Autodesk Inventor part; units mm, degrees
ref_plane "YZ Plane" through (0, 0, 0) normal (1, 0, 0) x (0, 1, 0)
ref_plane "XZ Plane" through (0, 0, 0) normal (0, 1, 0) x (-1, 0, 0)
ref_plane "XY Plane" through (0, 0, 0) normal (0, 0, 1) x (1, 0, 0)
sketch "Sketch1" plane through (0, 0, 0) normal (0, 0, 1) x (1, 0, 0)
  circle A0 centre (0, 0) radius 4
  line L0 (-10, -10) -> (10, -10)
  line L1 (10, -10) -> (10, 10)
  line L2 (10, 10) -> (-10, 10)
  line L3 (-10, 10) -> (-10, -10)
  line L4 (-10, -10) -> (10, 10) construction
  line L5 (10, -10) -> (-10, 10) construction
  dimension "d0" = 8
  dimension "d3" = 20
  dimension "d4" = 10
  dimension "d5" = 10
extrude "Extrusion1" add sketch "Sketch1" along normal blind 30 and the other way blind 20
extrude "Extrusion2" add sketch "Sketch1" against normal up to surface (20 mm away) contours A0
sketch "Sketch2" plane through (-10, -10, 30) normal (-1, 0, 0) x (0, 0, 1)
  line L0 (-50, 20) -> (-50, 0)
  line L1 (-50, 20) -> (-30, 20)
  line L2 (-30, 20) -> (-30, 0)
  line L3 (-30, 0) -> (-50, 0)
  line L4 (-50, 0) -> (-50, 20)
  point P0 (-30, 10)
extrude "Extrusion3" add sketch "Sketch2" along normal blind 30
sketch "Sketch3" plane through (-10, -10, 30) normal (0, -1, 0) x (1, 0, 0)
  line L0 (0, -30) -> (-30, -30)
  line L1 (0, -30) -> (20, -30)
  line L2 (20, -30) -> (20, -50)
  line L3 (20, -50) -> (0, -50)
  line L4 (0, -50) -> (0, -30)
  point P0 (10, -30)
extrude "Extrusion4" add sketch "Sketch3" along normal blind 30
sketch "Sketch4" plane through (-40, -10, 30) normal (-1, 0, 0) x (0, 0, 1)
  circle A0 centre (-40, 10) radius 4
  point P0 (-30, 10)
  dimension "d16" = 8
extrude "Extrusion5" cut sketch "Sketch4" against normal blind 30
sketch "Sketch5" plane through (-10, -40, 30) normal (0, -1, 0) x (1, 0, 0)
  circle A0 centre (10, -40) radius 4
  point P0 (10, -30)
  dimension "d19" = 8
extrude "Extrusion6" cut sketch "Sketch5" against normal blind 30
sketch "Sketch6" plane through (0, 0, -20) normal (0, 0, -1) x (-1, 0, 0)
  line L0 (10, -10) -> (40, -10)
  line L1 (10, -10) -> (10, -40)
  line L2 (10, -40) -> (-10, -40)
  line L3 (40, -10) -> (10, -40)
  point P0 (0, 0)
extrude "Extrusion7" add sketch "Sketch6" against normal blind 20
sketch "Sketch7" plane through (-10, 10, 30) normal (0, 1, 0) x (1, 0, 0)
  line L0 (-30, 30) -> (-30, 50)
  line L1 (0, 30) -> (-30, 30)
  line L2 (-30, 30) -> (0, 30)
  line L3 (0, 0) -> (20, 0)
  line L4 (0, 30) -> (0, 0)
  line L5 (0, 0) -> (-30, 30)
  point P0 (10, 30)
extrude "Extrusion8" add sketch "Sketch7" against normal blind 20
sketch "Sketch8" plane through (10, -10, 30) normal (1, 0, 0) x (0, 0, -1)
  line L0 (30, 0) -> (0, 0)
  line L1 (30, 0) -> (30, -30)
  line L2 (0, 20) -> (0, 0)
  line L3 (0, 0) -> (30, -30)
  point P0 (30, 10)
extrude "Extrusion9" add sketch "Sketch8" against normal blind 20
sketch "Sketch9" plane through (10, 10, 30) normal (0, 1, 0) x (1, 0, 0)
  line L0 (-50, 36) -> (-20, 36)
  line L1 (-14, 30) -> (-14, 0)
  circle A0 centre (-26.3015, 23.6985) radius 12.3015
  line L2 (-50, 30) -> (-20, 0)
  point P0 (-10, 30)
hole "Hole1" at (-16.3015, 10, 6.3015) direction (0, -1, 0) diameter 3.5 end through all
fillet "Fillet1" radius 4 3 edges at (-10, -25, 0) (-10, -10, 15) (-25, -10, 0)
fillet "Fillet2" radius 4 1 edges at (10, -15, -20)
fillet "Fillet3" radius 4 2 edges at (10, 0, 30) (-40, 0, -20)
move or copy body "Move Body1" bodies to move or copy 1 copy no rotation origin (0, 0, 0) rotation axis (-0.5773503, 0.5773503, -0.5773503) rotation angle 120 translate (30, 20, -10)
properties part number "connector" material "ABS Plastic"
The model under review builds one solid part; all positions refer to its coordinate system, in mm. A direction names the side the tool comes from. Round coordinates to 2 decimals unless told otherwise and drop trailing zeros. Loops run counter-clockwise (first coordinate to the right, second up) from the corner with the lowest first, then second, coordinate; pieces in that order, holes last. Notation, with made-up numbers: M -17,-5 L 5,-5 A23 cw 5,32 Z; hole C -39,44.5 d5. An arc over 180 degrees is marked long. Answer as a JSON object with one key per item and string values.
(1) Take a section at D-D on x = 20. Give the boundary of the cut face in (y, z), and give its area (3 significant figures).
Resolved:
{"outline": "M 10,-20 L 60,-20 L 60,-14 L 30,-14 L 30,-6 L 60,-6 L 60,0 L 30,30 L 24,30 L 24,0 L 16,0 L 16,30 L 10,30 Z", "area": "1,570 mm²"}
(2) Take a section at A-A on z = 24.5. Give the boundary of the cut face in (x, y).
Resolved:
{"outline": "M 10,14 A4 ccw 14,10 L 35.5,10 L 35.5,30 L 34,30 A4 cw 30,34 L 30,35.5 L 10,35.5 Z; hole C 20,20 d8"}
(3) Take a section at B-B on x = 36. Give the boundary of the cut face in (y, z), and give its area (3 significant figures).
Resolved:
{"outline": "M 10,-20 L 34.58,-20 L 34.58,0 L 34,0 A4 cw 30,4 L 30,24 L 10,24 Z; M 38.03,-20 L 54,-20 L 54,0 L 38.03,0 Z; hole C 20,-10 d8", "area": "1,240 mm²"}
(4) To check wall thickness, follow line 1 along Z through (x, y) = (46, 20); line 2 along Z through (x, y) = (37, 45); line 3 along Y through (x, z) = (42.5, 15.5). State the ranges of each line that lie inside material, in increasing order.
Resolved:
{"line 1": "-20 to -14, -6 to 14", "line 2": "-20 to 0", "line 3": "10 to 30"}
(5) Draft analysis for pull direction Z (two halves, no side actions). For faces 1 (the flat face through (10, 35, -1)), 2 (the cylindrical face through (46.24, 31.203, 1.141)), 3 (the flat face through (30, 20, -10)), 4 (the cylindrical face through (19.479, 45.21, -13.966)), state which applies: released by +Z, released by -Z, zero draft, split by the parting line, or undercut.
Resolved:
{"face 1": "zero draft", "face 2": "released by +Z", "face 3": "undercut", "face 4": "undercut"}
(6) Clearance check with flat-ended pins moving along their axes: P1, Ø8, axis at x = 46.5, y = 33, coming from the +Z side; P2, Ø3, axis at x = 36.3, y = 36.3, coming from the +Z side; P3, Ø11, axis at x = 45.5, y = 44, coming from the +Z side; P4, Ø6.5, axis at y = 46, z = 17.5, coming from the +X side. State where each tip first meets the part, or that it passes through.
Resolved:
{"P1": "z = 16.15", "P2": "through", "P3": "z = 0", "P4": "x = 30"}
(7) Tool access review of faces 5 (the flat face through (20, 30, -10)), 6 (the flat face through (20, 20, 0)), 7 (the flat face through (40, 30, 10)), 8 (the cylindrical face through (35.9, 34.6, -9.9)), 9 (the cylindrical face through (44.8, 23.2, -12.4)): name each direction out of +Z, -Z, +X, -X, +Y, -Y from which nothing blocks a thin tool from reaching the whole face with its end or side.
Resolved:
{"face 5": "+Y", "face 6": "+Z", "face 7": "+Z, +X, +Y", "face 8": "+Z, -Z", "face 9": "+X"}
(8) Take a section at C-C on y = 41. Give the boundary of the cut face in (x, z).
Resolved:
{"outline": "M 10,-20 L 49,-20 L 49,0 L 34,0 A4 cw 30,4 L 30,19 L 10,19 Z; hole C 20,-10 d8"}
